Read the model definition and answer for the solid it produces. Units are mm, in the model's axes. Face numbers are marked on the shaded views. A direction names the side the tool comes from. Round coordinates to 2 decimals unless told otherwise and drop trailing zeros. Order: outer loops, then holes, each group sorted by start corner. A loop starts at its lowest first (then second) coordinate and runs counter-clockwise, first axis right, second up. Notation, with made-up numbers: (70.25, 42.5) - (105.25, 42.5) arc R24 cw to (105.25, 62.5) - close; hole circle Ø2 at (74, -38). An arc over 180 degrees is marked (long way). Put each result on its own line as item: value. Start each with the question number.
Q1. Which of the six approach directions +Z, -Z, +X, -X, +Y, -Y give full straight-line access (tool end or side, diameter ignored) to the marked faces 5, 6 and 7?
Q2. Section C-C on x = 33 is taken. Give the vertices of the cut face in (y, z) (3 decimals), then the cut area to 3 significant figures.
Q3. For a pull along X with two mould halves and no side action, classify the marked faces 1, 2, 3 and 4 as pulls with the +X half, pulls with the -X half, needs draft (parallel to the pull), parting line crosses it, or undercut.
Q4. Section A-A on y = 0 is taken. State how many separate pieces and enclosed holes the cut face has, then the cut area to 3 significant figures.
Q5. Each of these flat-tipped pins is pushed along its axis until it touches: pin 1 Ø8 at (y, z) = (25, 35.5) entering from -X; pin 2 Ø21 at (x, z) = (-2, 8.5) entering from +Y (3 decimals); pin 3 Ø6 at (x, y) = (-12, -34) entering from -Z. Where does it stop, or does it pass through?
Q6. Find the intervals of material crossed by line 1 along X through (y, z) = (-17, 0) (3 decimals); line 2 along Z through (x, y) = (33, 0) (3 decimals), in increasing order. Write a range as from..to.
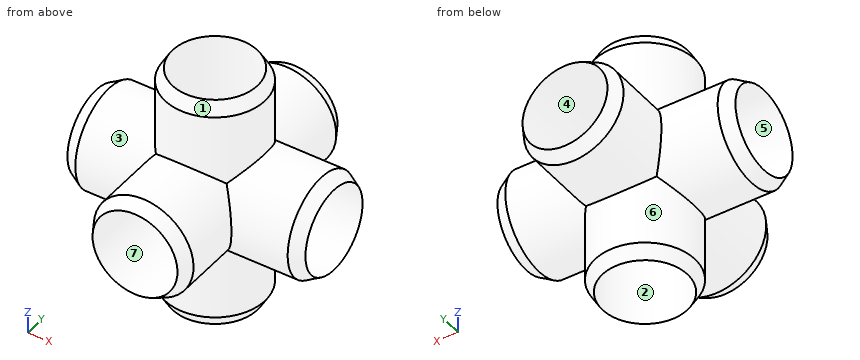
from build123d import *


with BuildPart() as f6:
    # F0 (on Right) → F6 (revolve)
    with BuildSketch(Plane.YZ):
        with BuildLine():
            Line((-52.6758568757, 24.765), (-59.055, 21.082))
            Line((-59.055, 21.082), (-20.955, 21.082))
            Line((-20.955, 21.082), (-20.955, 15.875))
            Line((-20.955, 15.875), (0, 15.875))
            ThreePointArc((0, 15.875), (11.2253201513, 11.2253201513), (15.875, 0))
            Line((15.875, 0), (24.765, 0))
            ThreePointArc((24.765, 0), (17.5114994361, 17.5114994361), (0, 24.765))
            Line((0, 24.765), (-52.6758568757, 24.765))
        make_face()
        with BuildLine():
            Line((-20.955, 21.082), (-59.055, 21.082))
            Line((-59.055, 21.082), (-59.055, 0))
            Line((-59.055, 0), (0, 0))
            Line((0, 0), (10.5189766587, 0))
            Line((10.5189766587, 0), (15.875, 0))
            ThreePointArc((15.875, 0), (11.2253201513, 11.2253201513), (0, 15.875))
            Line((0, 15.875), (-20.955, 15.875))
            Line((-20.955, 15.875), (-20.955, 21.082))
        make_face()
    revolve(axis=Axis((0, -21.59, 0), (0, 1, 0)))

    # F1 (on Right) → F7 (revolve)
    with BuildSketch(Plane.YZ):
        with BuildLine():
            Line((-24.765, -52.6758568757), (-21.082, -59.055))
            Line((-21.082, -59.055), (-21.082, -20.955))
            Line((-21.082, -20.955), (-15.875, -20.955))
            Line((-15.875, -20.955), (-15.875, 0))
            ThreePointArc((-15.875, 0), (-11.2253201513, 11.2253201513), (0, 15.875))
            Line((0, 15.875), (0, 24.765))
            ThreePointArc((0, 24.765), (-17.5114994361, 17.5114994361), (-24.765, 0))
            Line((-24.765, 0), (-24.765, -52.6758568757))
        make_face()
        with BuildLine():
            Line((-21.082, -20.955), (-21.082, -59.055))
            Line((-21.082, -59.055), (0, -59.055))
            Line((0, -59.055), (0, 0))
            Line((0, 0), (0, 15.875))
            ThreePointArc((0, 15.875), (-11.2253201513, 11.2253201513), (-15.875, 0))
            Line((-15.875, 0), (-15.875, -20.955))
            Line((-15.875, -20.955), (-21.082, -20.955))
        make_face()
    revolve(axis=Axis((0, 0, -21.59), (0, 0, 1)))

    # F2 (on Right) → F8 (revolve)
    with BuildSketch(Plane.YZ):
        with BuildLine():
            Line((52.6758568757, -24.765), (59.055, -21.082))
            Line((59.055, -21.082), (20.955, -21.082))
            Line((20.955, -21.082), (20.955, -15.875))
            Line((20.955, -15.875), (0, -15.875))
            ThreePointArc((0, -15.875), (-11.2253201513, -11.2253201513), (-15.875, 0))
            Line((-15.875, 0), (-24.765, 0))
            ThreePointArc((-24.765, 0), (-17.5114994361, -17.5114994361), (0, -24.765))
            Line((0, -24.765), (52.6758568757, -24.765))
        make_face()
        with BuildLine():
            Line((20.955, -21.082), (59.055, -21.082))
            Line((59.055, -21.082), (59.055, 0))
            Line((59.055, 0), (10.5189766587, 0))
            Line((10.5189766587, 0), (0, 0))
            Line((0, 0), (-15.875, 0))
            ThreePointArc((-15.875, 0), (-11.2253201513, -11.2253201513), (0, -15.875))
            Line((0, -15.875), (20.955, -15.875))
            Line((20.955, -15.875), (20.955, -21.082))
        make_face()
    revolve(axis=Axis((0, 21.59, 0), (0, -1, 0)))

    # F3 (on Right) → F9 (revolve)
    with BuildSketch(Plane.YZ):
        with BuildLine():
            Line((24.765, 52.6758568757), (21.082, 59.055))
            Line((21.082, 59.055), (21.082, 20.955))
            Line((21.082, 20.955), (15.875, 20.955))
            Line((15.875, 20.955), (15.875, 0))
            ThreePointArc((15.875, 0), (11.2253201513, -11.2253201513), (0, -15.875))
            Line((0, -15.875), (0, -24.765))
            ThreePointArc((0, -24.765), (17.5114994361, -17.5114994361), (24.765, 0))
            Line((24.765, 0), (24.765, 52.6758568757))
        make_face()
        with BuildLine():
            Line((21.082, 20.955), (21.082, 59.055))
            Line((21.082, 59.055), (0, 59.055))
            Line((0, 59.055), (0, 9.2996467855))
            Line((0, 9.2996467855), (0, 0))
            Line((0, 0), (0, -15.875))
            ThreePointArc((0, -15.875), (11.2253201513, -11.2253201513), (15.875, 0))
            Line((15.875, 0), (15.875, 20.955))
            Line((15.875, 20.955), (21.082, 20.955))
        make_face()
    revolve(axis=Axis((0, 0, 21.59), (0, 0, -1)))

    # F4 (on Top) → F10 (revolve)
    with BuildSketch(Plane.XY):
        with BuildLine():
            Line((-52.6758568757, 24.765), (-59.055, 21.082))
            Line((-59.055, 21.082), (-20.955, 21.082))
            Line((-20.955, 21.082), (-20.955, 15.875))
            Line((-20.955, 15.875), (0, 15.875))
            ThreePointArc((0, 15.875), (11.2253201513, 11.2253201513), (15.875, 0))
            Line((15.875, 0), (24.765, 0))
            ThreePointArc((24.765, 0), (17.5114994361, 17.5114994361), (0, 24.765))
            Line((0, 24.765), (-52.6758568757, 24.765))
        make_face()
        with BuildLine():
            Line((-20.955, 21.082), (-59.055, 21.082))
            Line((-59.055, 21.082), (-59.055, 0))
            Line((-59.055, 0), (-12.5608257832, 0))
            Line((-12.5608257832, 0), (0, 0))
            Line((0, 0), (15.875, 0))
            ThreePointArc((15.875, 0), (11.2253201513, 11.2253201513), (0, 15.875))
            Line((0, 15.875), (-20.955, 15.875))
            Line((-20.955, 15.875), (-20.955, 21.082))
        make_face()
    revolve(axis=Axis((-21.59, 0, 0), (1, 0, 0)))

    # F5 (on Top) → F11 (revolve)
    with BuildSketch(Plane.XY):
        with BuildLine():
            Line((52.6758568757, -24.765), (59.055, -21.082))
            Line((59.055, -21.082), (20.955, -21.082))
            Line((20.955, -21.082), (20.955, -15.875))
            Line((20.955, -15.875), (0, -15.875))
            ThreePointArc((0, -15.875), (-11.2253201513, -11.2253201513), (-15.875, 0))
            Line((-15.875, 0), (-24.765, 0))
            ThreePointArc((-24.765, 0), (-17.5114994361, -17.5114994361), (0, -24.765))
            Line((0, -24.765), (52.6758568757, -24.765))
        make_face()
        Polygon((20.955, -21.082), (59.055, -21.082), (59.055, 0), (30.3153488902, 0), (0, 0), (0, -15.875), (20.955, -15.875), align=None)
        with BuildLine():
            ThreePointArc((-15.875, 0), (-11.2253201513, -11.2253201513), (0, -15.875))
            Line((0, -15.875), (0, 0))
            Line((0, 0), (-15.875, 0))
        make_face()
    revolve(axis=Axis((21.59, 0, 0), (-1, 0, 0)))

    # F0 (on Right) → F12 (revolve, cut)
    with BuildSketch(Plane.YZ):
        with BuildLine():
            Line((-20.955, 21.082), (-59.055, 21.082))
            Line((-59.055, 21.082), (-59.055, 0))
            Line((-59.055, 0), (0, 0))
            Line((0, 0), (10.5189766587, 0))
            Line((10.5189766587, 0), (15.875, 0))
            ThreePointArc((15.875, 0), (11.2253201513, 11.2253201513), (0, 15.875))
            Line((0, 15.875), (-20.955, 15.875))
            Line((-20.955, 15.875), (-20.955, 21.082))
        make_face()
    revolve(axis=Axis((0, -21.59, 0), (0, 1, 0)), mode=Mode.SUBTRACT)

    # F1 (on Right) → F13 (revolve, cut)
    with BuildSketch(Plane.YZ):
        with BuildLine():
            Line((-21.082, -20.955), (-21.082, -59.055))
            Line((-21.082, -59.055), (0, -59.055))
            Line((0, -59.055), (0, 0))
            Line((0, 0), (0, 15.875))
            ThreePointArc((0, 15.875), (-11.2253201513, 11.2253201513), (-15.875, 0))
            Line((-15.875, 0), (-15.875, -20.955))
            Line((-15.875, -20.955), (-21.082, -20.955))
        make_face()
    revolve(axis=Axis((0, 0, -21.59), (0, 0, 1)), mode=Mode.SUBTRACT)

    # F2 (on Right) → F14 (revolve, cut)
    with BuildSketch(Plane.YZ):
        with BuildLine():
            Line((20.955, -21.082), (59.055, -21.082))
            Line((59.055, -21.082), (59.055, 0))
            Line((59.055, 0), (10.5189766587, 0))
            Line((10.5189766587, 0), (0, 0))
            Line((0, 0), (-15.875, 0))
            ThreePointArc((-15.875, 0), (-11.2253201513, -11.2253201513), (0, -15.875))
            Line((0, -15.875), (20.955, -15.875))
            Line((20.955, -15.875), (20.955, -21.082))
        make_face()
    revolve(axis=Axis((0, 21.59, 0), (0, -1, 0)), mode=Mode.SUBTRACT)

    # F3 (on Right) → F15 (revolve, cut)
    with BuildSketch(Plane.YZ):
        with BuildLine():
            Line((21.082, 20.955), (21.082, 59.055))
            Line((21.082, 59.055), (0, 59.055))
            Line((0, 59.055), (0, 9.2996467855))
            Line((0, 9.2996467855), (0, 0))
            Line((0, 0), (0, -15.875))
            ThreePointArc((0, -15.875), (11.2253201513, -11.2253201513), (15.875, 0))
            Line((15.875, 0), (15.875, 20.955))
            Line((15.875, 20.955), (21.082, 20.955))
        make_face()
    revolve(axis=Axis((0, 0, 21.59), (0, 0, -1)), mode=Mode.SUBTRACT)

    # F4 (on Top) → F16 (revolve, cut)
    with BuildSketch(Plane.XY):
        with BuildLine():
            Line((-20.955, 21.082), (-59.055, 21.082))
            Line((-59.055, 21.082), (-59.055, 0))
            Line((-59.055, 0), (-12.5608257832, 0))
            Line((-12.5608257832, 0), (0, 0))
            Line((0, 0), (15.875, 0))
            ThreePointArc((15.875, 0), (11.2253201513, 11.2253201513), (0, 15.875))
            Line((0, 15.875), (-20.955, 15.875))
            Line((-20.955, 15.875), (-20.955, 21.082))
        make_face()
    revolve(axis=Axis((-21.59, 0, 0), (1, 0, 0)), mode=Mode.SUBTRACT)

    # F5 (on Top) → F17 (revolve, cut)
    with BuildSketch(Plane.XY):
        Polygon((20.955, -21.082), (59.055, -21.082), (59.055, 0), (30.3153488902, 0), (0, 0), (0, -15.875), (20.955, -15.875), align=None)
    revolve(axis=Axis((21.59, 0, 0), (-1, 0, 0)), mode=Mode.SUBTRACT)


solid = f6.part
Findings:
1. face 5: -X
1. face 6: -Z
1. face 7: -Y
2. outline: circle Ø49.53 at (0, 0); hole circle Ø42.164 at (0, 0)
2. area: 530 mm2
3. face 1: parting line crosses it
3. face 2: undercut
3. face 3: needs draft
3. face 4: undercut
4. separate pieces: 8
4. enclosed holes: 0
4. area: 1,070 mm2
5. pin 1: x = -13.13
5. pin 2: y = 20.955
5. pin 3: z = -23.07
6. line 1: -20.955..-15.875, 15.875..20.955
6. line 2: -24.765..-21.082, 21.082..24.765
